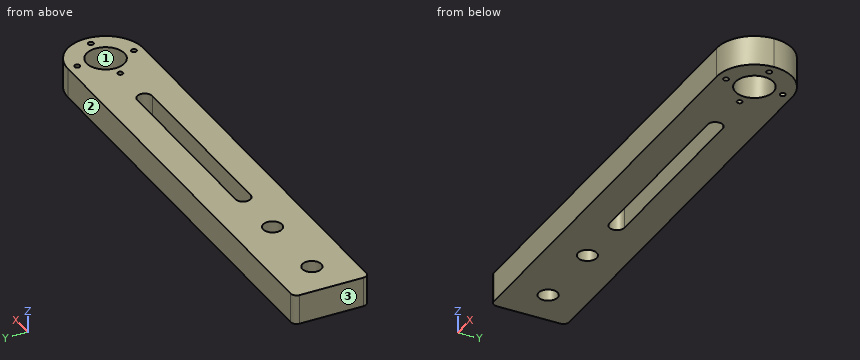
from build123d import *

# Parameters (mm, degrees)
SKETCH1_R           = 3.175
SKETCH1_R_2         = 6.35
SKETCH1_R_3         = 0.9
BOSS_EXTRUDE1_DEPTH = 10
FILLET2_R           = 2
FILLET3_R           = 12.7


with BuildPart() as part:
    # Sketch1 → Boss-Extrude1 (new body)
    with BuildSketch(Plane.XY):
        Polygon((-73.025, -12.7), (-73.025, 12.7), (73.025, 12.7), (85.725, 12.7), (85.725, -12.7), (73.025, -12.7), align=None)
        with Locations((-60.325, 0)):
            Circle(SKETCH1_R, mode=Mode.SUBTRACT)
        with Locations((73.025, 0)):
            Circle(SKETCH1_R_2, mode=Mode.SUBTRACT)
        with Locations((73.025, 9.525)):
            Circle(SKETCH1_R_3, mode=Mode.SUBTRACT)
        with Locations((73.025, -9.525)):
            Circle(SKETCH1_R_3, mode=Mode.SUBTRACT)
        with Locations((63.5, 0)):
            Circle(SKETCH1_R_3, mode=Mode.SUBTRACT)
        with Locations((82.55, 0)):
            Circle(SKETCH1_R_3, mode=Mode.SUBTRACT)
        with Locations((-34.925, 0)):
            Circle(SKETCH1_R, mode=Mode.SUBTRACT)
        with BuildLine():
            Line((-15.875, 2.54), (47.625, 2.54))
            ThreePointArc((47.625, 2.54), (50.165, 0), (47.625, -2.54))
            Line((47.625, -2.54), (-15.875, -2.54))
            ThreePointArc((-15.875, -2.54), (-18.415, 0), (-15.875, 2.54))
        make_face(mode=Mode.SUBTRACT)
    extrude(amount=BOSS_EXTRUDE1_DEPTH)

    # Fillet2
    fillet2_edges = [part.edges().sort_by_distance(p)[0] for p in [
        (-73.025, -12.7, 5),
        (-73.025, 12.7, 5),
    ]]
    fillet(fillet2_edges, radius=FILLET2_R)

    # Fillet3
    fillet3_edges = [part.edges().sort_by_distance(p)[0] for p in [
        (85.725, 12.7, 5),
        (85.725, -12.7, 5),
    ]]
    fillet(fillet3_edges, radius=FILLET3_R - 0.0001)  # a hair under: the kernel refuses the full size


solid = part.part
Design review of the part built by this model. Coordinates are the model's own, in mm. Face numbers are marked on the shaded views. Coordinates: 2 decimals unless noted, no trailing zeros. Write each loop counter-clockwise with the first axis right and the second up, starting at its lowest first coordinate (ties: lowest second). Pieces come first, ordered by that corner, then holes. Notation, with made-up numbers: (18.25, 43) -> (60.25, 43) arc R20 cw to (60.25, 59) -> close; hole circle Ø6 at (-39.75, -1.75). An arc over 180 degrees is marked (long way). Write each question's results on one line, items separated by ' | '. Start each with the question number.
(1) Clearance check with a flat-ended pin moving along its axis: P1, Ø14.5, axis at x = 73.025, y = 0, coming from the +Z side. State where the tip first meets the part, or that it passes through.
(2) Take a section at B-B on z = 6.25. Give the number of separate pieces and of enclosed holes in the cut face, and give its area (3 significant figures).
(3) For line 1 along Y through (x, z) = (5, 5.5); line 2 along Y through (x, z) = (63.5, 2); line 3 along X through (y, z) = (-7.25, 8.75) (3 decimals), list the stretches that pass through material, from the lowest coordinate up. Write a range as from..to.
(4) Take a section at C-C on x = -36. Write out the cut boundary in (y, z).
(5) Take a section at A-A on x = -4. Write out the cut boundary in (y, z), and give its area (3 significant figures).
(6) The part is to be moulded in two halves that separate along Y. For the marked faces 1, 2 and 3, say which applies: pulls with the +Y half, pulls with the -Y half, needs draft (parallel to the pull), parting line crosses it, or undercut.
Results found:
1) P1: stops at z = 10
2) separate pieces: 1 | enclosed holes: 8 | area: 3,420 mm2
3) line 1: y = -12.7..-2.54, 2.54..12.7 | line 2: y = -12.7..-0.9, 0.9..12.7 | line 3: x = -73.025..83.452
4) outline: (-12.7, 0) -> (-2.99, 0) -> (-2.99, 10) -> (-12.7, 10) -> close; (2.99, 0) -> (12.7, 0) -> (12.7, 10) -> (2.99, 10) -> close
5) outline: (-12.7, 0) -> (-2.54, 0) -> (-2.54, 10) -> (-12.7, 10) -> close; (2.54, 0) -> (12.7, 0) -> (12.7, 10) -> (2.54, 10) -> close | area: 203 mm2
6) face 1: undercut | face 2: pulls with the +Y half | face 3: needs draft
